The listing builds one solid part. Answer for the finished solid, in the listing's coordinates (mm). Face numbers are marked on the shaded views. A direction names the side the tool comes from. Give positions to 0.01 mm unless a question says otherwise; leave off trailing zeros. Order: outer loops, then holes, each group sorted by start corner. A loop starts at its lowest first (then second) coordinate and runs counter-clockwise, first axis right, second up. Notation, with made-up numbers: (45, 10.5) - (92, 10.5) arc R28 cw to (92, 43.5) - close; hole circle Ø11 at (64.5, -13). An arc over 180 degrees is marked (long way). Write each question's results on one line, items separated by ' | '. Start each with the question number.
1. Section C-C (z = 1.25) is taken. Give the vertices of the cut face in (x, y), and give its area (3 significant figures).
2. Section A-A (y = 0) is taken. Give the vertices of the cut face in (x, z).
3. Find the intervals of material crossed by L1, parallel to Z at x = 6, y = -10.5; L2, parallel to Z at x = 16, y = 10.5; L3, parallel to Y at x = -13.5, z = 1, in increasing order.
4. Which of the six approach directions +Z, -Z, +X, -X, +Y, -Y give full straight-line access (tool end or side, diameter ignored) to the marked faces 1 and 2?
5. Flat-ended cylindrical pins translate along their axes: pin 1 (10 mm diameter, centred on x = -15, y = 9.5, fed in from +Z); pin 2 (2 mm diameter, centred on y = -10, z = 0.5, fed in from -X); pin 3 (1 mm diameter, centred on y = 3.5, z = 1.5, fed in from +X). Find the tip coordinate at first contact, or state that the pin passes through.
6. Section B-B (x = 9) is taken. Give the vertices of the cut face in (y, z), and give its area (3 significant figures).
from build123d import *

# Parameters (mm, degrees)
SKETCH1_R           = 25
SKETCH1_R_2         = 22.5
SKETCH1_R_3         = 15
SKETCH1_R_4         = 7.5
BOSS_EXTRUDE1_DEPTH = 2
BOSS_EXTRUDE2_START = 2
SKETCH1_3_R         = 22.5
SKETCH1_3_R_2       = 15
SKETCH1_3_R_3       = 7.5
BOSS_EXTRUDE2_DEPTH = 1
BOSS_EXTRUDE3_START = 3
SKETCH1_4_R         = 15
SKETCH1_4_R_2       = 7.5
BOSS_EXTRUDE3_DEPTH = 0.5
BOSS_EXTRUDE4_START = 3.5
SKETCH1_5_R         = 7.5
BOSS_EXTRUDE4_DEPTH = 3


with BuildPart() as part:
    # Sketch1 → Boss-Extrude1 (new body)
    # profile 1 of 4: a face of its own
    with BuildSketch(Plane.XY):
        Circle(SKETCH1_R)
        Circle(SKETCH1_R_2, mode=Mode.SUBTRACT)
    # profile 2 of 4: a face of its own
    with BuildSketch(Plane.XY):
        Circle(SKETCH1_R_2)
        Circle(SKETCH1_R_3, mode=Mode.SUBTRACT)
    # profile 3 of 4: a face of its own
    with BuildSketch(Plane.XY):
        Circle(SKETCH1_R_3)
        Circle(SKETCH1_R_4, mode=Mode.SUBTRACT)
    # profile 4 of 4: a face of its own
    with BuildSketch(Plane.XY):
        Circle(SKETCH1_R_4)
    extrude(amount=BOSS_EXTRUDE1_DEPTH)

    # Sketch1<3> → Boss-Extrude2 (add)
    # profile 1 of 3: a face of its own
    with BuildSketch(Plane.XY.offset(BOSS_EXTRUDE2_START)):
        Circle(SKETCH1_3_R)
        Circle(SKETCH1_3_R_2, mode=Mode.SUBTRACT)
    # profile 2 of 3: a face of its own
    with BuildSketch(Plane.XY.offset(BOSS_EXTRUDE2_START)):
        Circle(SKETCH1_3_R_2)
        Circle(SKETCH1_3_R_3, mode=Mode.SUBTRACT)
    # profile 3 of 3: a face of its own
    with BuildSketch(Plane.XY.offset(BOSS_EXTRUDE2_START)):
        Circle(SKETCH1_3_R_3)
    extrude(amount=BOSS_EXTRUDE2_DEPTH)

    # Sketch1<4> → Boss-Extrude3 (add)
    # profile 1 of 2: a face of its own
    with BuildSketch(Plane.XY.offset(BOSS_EXTRUDE3_START)):
        Circle(SKETCH1_4_R)
        Circle(SKETCH1_4_R_2, mode=Mode.SUBTRACT)
    # profile 2 of 2: a face of its own
    with BuildSketch(Plane.XY.offset(BOSS_EXTRUDE3_START)):
        Circle(SKETCH1_4_R_2)
    extrude(amount=BOSS_EXTRUDE3_DEPTH)

    # Sketch1<5> → Boss-Extrude4 (add)
    with BuildSketch(Plane.XY.offset(BOSS_EXTRUDE4_START)):
        Circle(SKETCH1_5_R)
    extrude(amount=BOSS_EXTRUDE4_DEPTH)


solid = part.part
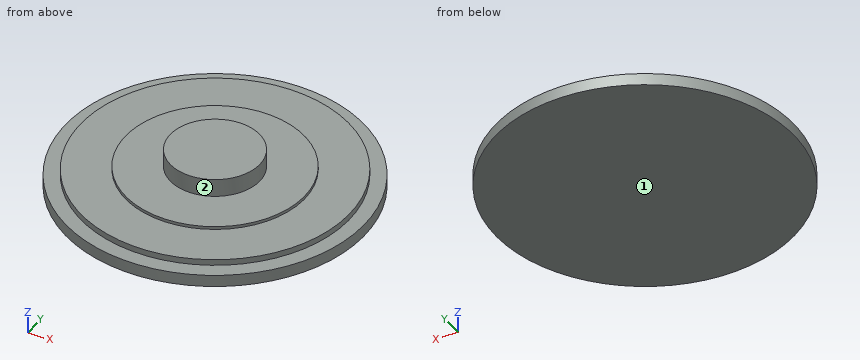
Reported:
1) outline: circle Ø50 at (0, 0) | area: 1,960 mm²
2) outline: (-25, 0) - (25, 0) - (25, 2) - (22.5, 2) - (22.5, 3) - (15, 3) - (15, 3.5) - (7.5, 3.5) - (7.5, 6.5) - (-7.5, 6.5) - (-7.5, 3.5) - (-15, 3.5) - (-15, 3) - (-22.5, 3) - (-22.5, 2) - (-25, 2) - close
3) L1: 0 to 3.5 | L2: 0 to 3 | L3: -21.04 to 21.04
4) face 1: -Z, +X, -X, +Y, -Y | face 2: +Z
5) pin 1: z = 3.5 | pin 2: x = -23.32 | pin 3: x = 24.82
6) outline: (-23.32, 0) - (23.32, 0) - (23.32, 2) - (20.62, 2) - (20.62, 3) - (12, 3) - (12, 3.5) - (-12, 3.5) - (-12, 3) - (-20.62, 3) - (-20.62, 2) - (-23.32, 2) - close | area: 147 mm²
